Can you work these out from the model? Positions are in its coordinate system, mm. Face numbers are marked on the shaded views. A direction names the side the tool comes from. Round coordinates to 2 decimals unless told otherwise and drop trailing zeros. Write each loop counter-clockwise with the first axis right and the second up, starting at its lowest first coordinate (ties: lowest second). Pieces come first, ordered by that corner, then holes. Notation, with made-up numbers: (77.25, 51) -> (117.25, 51) arc R12 cw to (117.25, 59) -> close; hole circle Ø2 at (72, 14). An arc over 180 degrees is marked (long way). Write item = value, one per line. Start each with the question number.
1) Imagine slicing it at B-B, the plane x = -6. Please give me the cut outline in (y, z), then the cut area to 3 significant figures.
2) Imagine slicing it at A-A, the plane y = -3.5. Please give me the cut outline in (x, z), then the cut area to 3 significant figures.
3) If I drill on line 1 (X direction, y = -12.5, z = 0); line 2 (Z direction, x = 1, y = -33); line 3 (X direction, y = -20.5, z = -8), over which ranges is the centre line in solid material (lowest first)?
4) I'm going to push flat-ended pins straight in: pin 1 (5 mm diameter, centred on y = -27.5, z = -15, fed in from -X); pin 2 (6 mm diameter, centred on y = -30, z = 14, fed in from -X); pin 3 (1 mm diameter, centred on x = -38, y = -25, fed in from -Z). Where does each tip first touch, or does it pass through?
5) Imagine slicing it at D-D, the plane z = -5. Please give me the cut outline in (x, y).
6) Thinking about a two-plate mould opening in Z: for the marked faces 4, 5 and 6, which applies, +Z half, -Z half, draft (parallel to the pull), parting line (faces both ways), or undercut?
7) For the marked faces 1, 2 and 3, which set-ups out of +Z, -Z, +X, -X, +Y, -Y let a thin tool reach every point of the face, with its end or its side?
8) Imagine slicing it at C-C, the plane y = -17. Please give me the cut outline in (x, z) (1 decimal), then the cut area to 3 significant figures.
Autodesk Inventor part; units mm, degrees
ref_plane "Work Plane1" through (0, -5, 0) normal (0, -1, 0) x (1, 0, 0)
ref_plane "Work Plane2" through (0, -35, 0) normal (0, -1, 0) x (1, 0, 0)
ref_plane "YZ Plane" through (0, 0, 0) normal (1, 0, 0) x (0, 1, 0)
sketch "Sketch1" plane through (0, 0, 0) normal (0, 1, 0) x (-1, 0, 0)
  line L0 (30, 0) -> (-30, 0) construction
  line L1 (30, 25) -> (-30, 25) construction
  line L2 (-30, -25) -> (30, -25)
  arc A0 (30, -25) -> (30, 25) centre (30, 0) ccw construction
  arc A1 (-30, 25) -> (-30, -25) centre (-30, 0) ccw
  line L3 (30, -25) -> (0, 0) construction
  line L4 (0, 0) -> (30, 25) construction
  line L5 (0, 0) -> (-34.4376, -24.603) construction
  line L6 (0, 0) -> (-34.4376, 25) construction
  line L7 (-34.4376, -24.603) -> (-34.4376, 25) construction
  line L8 (30, -25) -> (30, 25) construction
  line L9 (55, 0) -> (30, -25) construction
  line L10 (55, 0) -> (30, 25) construction
  line L11 (-34.4376, -24.603) -> (-55, 0) construction
  line L12 (-55, 0) -> (-30, 25) construction
  line L13 (25, 0) -> (-25, 0) construction
  line L14 (25, 25) -> (-25, 25) construction
  line L15 (-25, -25) -> (25, -25) construction
  arc A2 (25, -25) -> (25, 25) centre (25, 0) ccw construction
  arc A3 (-25, 25) -> (-25, -25) centre (-25, 0) ccw construction
  line L16 (55, 0) -> (25, -25) construction
  line L17 (55, 0) -> (25, 25) construction
  line L18 (25, -25) -> (25, 25) construction
  line L19 (0, 0) -> (55, 0) construction
  line L20 (-25, -25) -> (-25, 25) construction
  circle A4 centre (-30, 0) radius 25 construction
  circle A5 centre (30, 0) radius 25 construction
  circle A6 centre (-30, 0) radius 22.5 construction
  line L21 (30, -25) -> (-30, -25)
  line L22 (0, -25) -> (0, 25) construction
  line L23 (30, 0) -> (0, 25) construction
  line L24 (10.7945, 16.0046) -> (-10.7945, 16.0046) construction
  line L25 (10.7945, 16.0046) -> (-10.7945, 16.0046)
  line L26 (8.9613, 13.5046) -> (-8.9613, 13.5046)
  circle A7 centre (30, 0) radius 10
  line L27 (19.1028, -22.5) -> (-19.1028, -22.5)
  line L28 (-30, 0) -> (-30, -25) construction
  line L29 (-30, 0) -> (-30, 25) construction
  line L30 (-30, 0) -> (-12.3223, -17.6777) construction
  line L31 (-30, 0) -> (-47.6777, -17.6777) construction
  line L32 (-25, -5) -> (-34.4376, -5) construction
  line L33 (-12.3223, -17.6777) -> (-47.6777, 17.6777) construction
  line L34 (-47.6777, -17.6777) -> (-12.3223, 17.6777) construction
  line L35 (-25, 5) -> (-34.4376, 5) construction
  circle A8 centre (-30, -5) radius 1.25
  circle A9 centre (-25, 0) radius 1.25
  circle A10 centre (-34.4376, 0) radius 1.25
  circle A11 centre (-30, 5) radius 1.25
  line L36 (-19.1028, -22.5) -> (-19.1028, 22.5) construction
  line L37 (19.1028, -22.5) -> (19.0552, 22.4769) construction
  line L38 (10.7945, 16.0046) -> (10.7945, -22.5636) construction
  line L39 (10.7945, 16.0046) -> (49.3627, 16.0046) construction
  line L40 (-10.7945, 16.0046) -> (-10.7945, -22.0758) construction
  line L41 (-10.7945, 16.0046) -> (27.2859, 16.0046) construction
  line L42 (-10.7945, -22.0758) -> (-11.3044, -22.5) construction
  line L43 (-8.9613, 13.5046) -> (-8.9613, -22.5) construction
  line L44 (8.9613, 13.5046) -> (8.9613, -22.5) construction
  arc A12 (19.0998, -19.6834) -> (30, -22.5) centre (30, 0) ccw
  arc A13 (30, -22.5) -> (52.5, 0) centre (30, 0) ccw
  arc A14 (52.5, 0) -> (30, 22.5) centre (30, 0) ccw
  arc A15 (39.375, 20.4538) -> (19.0582, 19.6603) centre (30, 0) ccw
  circle A16 centre (30, 0) radius 22.5369 construction
  arc A17 (19.0582, 19.6603) -> (11.9574, 13.5046) centre (29.9457, -0.0723) ccw
  line L45 (8.9613, 13.5046) -> (11.9574, 13.5046)
  line L46 (19.0998, -19.6834) -> (19.1028, -22.5)
  arc A18 (30, 25) -> (10.7945, 16.0046) centre (30, 0) ccw
  arc A19 (55, 0) -> (30, 25) centre (30, 0) ccw
  arc A20 (30, -25) -> (55, 0) centre (30, 0) ccw
  arc A21 (-52.4985, -0.2589) -> (-19.1028, -19.685) centre (-30, 0) ccw
  arc A22 (-19.1028, 19.685) -> (-52.4985, -0.2589) centre (-30, 0) ccw
  line L47 (-8.9613, 13.5046) -> (-12.0035, 13.5046)
  arc A23 (-12.0035, 13.5046) -> (-19.1028, 19.685) centre (-30, 0) ccw
  line L48 (-19.1028, -22.5) -> (-19.1028, -19.685)
  arc A24 (-10.7945, 16.0046) -> (-30, 25) centre (-30, 0) ccw
  point P0 (-30, 25)
  point P1 (-30, 0)
  dimension "d1" = 30
  dimension "d2" = 50
  dimension "d3" = 50
  dimension "d4" = 25
  dimension "d8" = 110
  dimension "d9" = 50
  dimension "d12" = 45
  dimension "d13" = 0
  dimension "d14" = 2.5
  dimension "d15" = 20
  dimension "d16" = 2.5
  dimension "d25" = 2.5
  dimension "d26" = 2.5
  dimension "d27" = 2.5
  dimension "d28" = 2.5
  dimension "d29" = 90
  dimension "d30" = 90
ref_plane "Work Plane1" through (0, -5, 0) normal (0, -1, 0) x (1, 0, 0)
extrude "Extrusion2" add sketch "Sketch1" against normal blind 35 contours A1 A24 L25 A18 A19 A20 L2
extrude "Extrusion3" add sketch "Sketch1" against normal blind 5 contours L45 A17 A15 A14 A13 A12 L46 L27 L48 A21 A22 A23 L47 L26
sketch "Sketch3" plane through (0, -35, 0) normal (0, -1, 0) x (1, 0, 0)
  point P0 (0, 0)
ref_plane "Work Plane2" through (0, -35, 0) normal (0, -1, 0) x (1, 0, 0)
sketch "Sketch4" plane through (0, -35, 0) normal (0, -1, 0) x (1, 0, 0)
  line L0 (0, 0) -> (-55, 0) construction
  arc A0 (-10.7945, 16.0046) -> (-30, -25) centre (-30, 0) ccw construction
  arc A1 (30, -25) -> (10.7945, 16.0046) centre (30, 0) ccw construction
  line L1 (0, 0) -> (55, 0) construction
  line L2 (-30, -25) -> (-30, 25) construction
  line L3 (30, -25) -> (30, 25) construction
  line L4 (-30, 13.5046) -> (30, 13.5046) construction
  line L5 (-19.1028, -22.5) -> (-19.0998, -19.6834) construction
  line L6 (-19.0998, -19.6834) -> (-30, -19.6834) construction
  arc A2 (-19.0582, 19.6603) -> (-19.0998, -19.6834) centre (-30, 0) ccw construction
  line L7 (-19.0998, -19.6834) -> (30, -19.6834) construction
  circle A3 centre (-53.8, 0) radius 0.75
  circle A4 centre (53.8, 0) radius 0.75
  arc A5 (19.1028, -19.685) -> (12.0035, 13.5046) centre (30, 0) ccw construction
  line L8 (-10.7945, 16.0046) -> (-10.7945, 13.5046) construction
  line L9 (10.7945, 16.0046) -> (10.7945, 13.5046) construction
  circle A6 centre (-10.7945, 14.7546) radius 0.75
  circle A7 centre (10.7945, 14.7546) radius 0.75
  point P0 (-52.5, 0.0238)
  point P1 (-52.5, 0.0238)
  dimension "d41" = 2.5
  dimension "d42" = 1.5
  dimension "d43" = 1.3
  dimension "d44" = 1.5
  dimension "d45" = 0.55
  dimension "d46" = 1.5
  dimension "d47" = 1.5
  dimension "d48" = 20.0889
extrude "Extrusion4" cut sketch "Sketch4" against normal blind 5
properties part number "con_v6_d1_3DPrint"
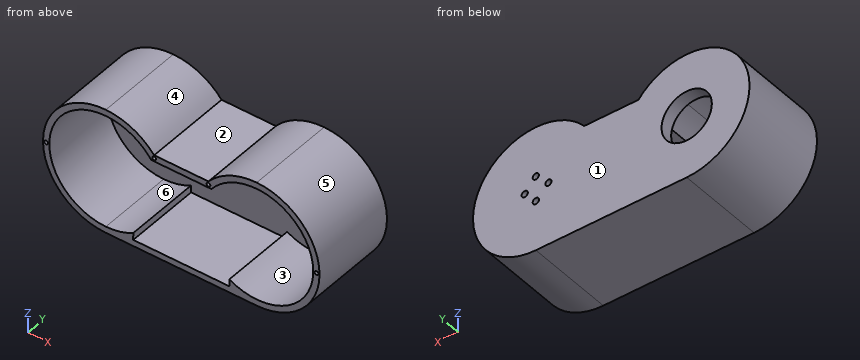
Reported:
q1.outline = (-35, -25) -> (0, -25) -> (0, 16) -> (-35, 16) -> (-35, 13.5) -> (-5, 13.5) -> (-5, -22.5) -> (-35, -22.5) -> close
q1.area = 355 mm²
q2.outline = (-30, -25) -> (30, -25) arc R25 ccw to (30, 25) arc R25 ccw to (10.79, 16) -> (-10.79, 16) arc R25 ccw to (-30, 25) arc R25 ccw to start; hole circle Ø20 at (-30, 0); hole circle Ø2.5 at (25, 0); hole circle Ø2.5 at (30, -5); hole circle Ø2.5 at (30, 5); hole circle Ø2.5 at (34.44, 0)
q2.area = 4,330 mm²
q3.line_1 = -55 to -52.5, 52.5 to 55
q3.line_2 = -25 to -22.5, 13.5 to 16
q3.line_3 = -53.69 to -51.03, 51.03 to 53.69
q4.pin_1 = -51.65
q4.pin_2 = -52.45
q4.pin_3 = -23.85
q5.outline = (-54.49, -35) -> (-51.94, -35) -> (-51.94, -5) -> (-38.66, -5) -> (-38.66, 0) -> (-54.49, 0) -> close; (-21.34, -5) -> (28.75, -5) -> (28.75, 0) -> (-21.34, 0) -> close; (31.25, -5) -> (51.94, -5) -> (51.94, -35) -> (54.49, -35) -> (54.49, 0) -> (31.25, 0) -> close
q6.face_4 = +Z half
q6.face_5 = parting line
q6.face_6 = undercut
q7.face_1 = +Z, -Z, +X, -X, +Y
q7.face_2 = +Z, +Y, -Y
q7.face_3 = -Y
q8.outline = (-30, -25) -> (30, -25) arc R25 ccw to (30, 25) arc R25 ccw to (10.8, 16) -> (-10.8, 16) arc R25 ccw to (-30, 25) arc R25 ccw to start; hole (-30, -22.5) arc R22.5 ccw to (-19.1, -19.7) -> (-19.1, -22.5) -> (19.1, -22.5) -> (19.1, -19.7) arc R22.5 ccw to (52.5, -0.3) arc R22.5 ccw to (19.1, 19.7) arc R22.5 ccw to (12, 13.5) -> (-12, 13.5) arc R22.5 ccw to (-19.1, 19.7) arc R22.5 ccw to (-30, 22.5) arc R22.5 ccw to start
q8.area = 707 mm²
